from build123d import *

# Parameters (mm, degrees)
CYLINDER016_R     = 0.5
CYLINDER016_DEPTH = 10
CYLINDER014_R     = 2
CYLINDER014_DEPTH = 4
CYLINDER015_R     = 3
CYLINDER015_DEPTH = 10
BOX003_W          = 10
BOX003_H          = 10
BOX003_DEPTH      = 10
BOX004_W          = 2
BOX004_H          = 10
BOX004_DEPTH      = 10
BOX002_W          = 10
BOX002_H          = 10
BOX002_DEPTH      = 10
CYLINDER013_R     = 5
CYLINDER013_DEPTH = 10
CYLINDER012_R     = 5
CYLINDER012_DEPTH = 10


with BuildPart() as cylinder016:
    # Cylinder016 → Cylinder016 (new body)
    with BuildSketch(Plane(origin=(-5, 0, -7), x_dir=(0, 0, -1), z_dir=(1, 0, 0))):
        Circle(CYLINDER016_R)
    extrude(amount=CYLINDER016_DEPTH)


with BuildPart() as cylinder014:
    # Cylinder014 → Cylinder014 (new body)
    with BuildSketch(Plane(origin=(-2, -50, 1), x_dir=(0, 0, -1), z_dir=(1, 0, 0))):
        Circle(CYLINDER014_R)
    extrude(amount=CYLINDER014_DEPTH)


with BuildPart() as cylinder015:
    # Cylinder015 → Cylinder015 (new body)
    with BuildSketch(Plane(origin=(0, -50, -12), x_dir=(1, 0, 0), z_dir=(0, 0, 1))):
        Circle(CYLINDER015_R)
    extrude(amount=CYLINDER015_DEPTH)


with BuildPart() as cube003:
    # Box003 → Box003 (new body)
    with BuildSketch(Plane(origin=(-12, -55, -2), x_dir=(1, 0, 0), z_dir=(0, 0, 1))):
        with Locations((5, 5)):
            Rectangle(BOX003_W, BOX003_H)
    extrude(amount=BOX003_DEPTH)


with BuildPart() as cube004:
    # Box004 → Box004 (new body)
    with BuildSketch(Plane(origin=(-1, -55, -2), x_dir=(1, 0, 0), z_dir=(0, 0, 1))):
        with Locations((1, 5)):
            Rectangle(BOX004_W, BOX004_H)
    extrude(amount=BOX004_DEPTH)


with BuildPart() as cube002:
    # Box002 → Box002 (new body)
    with BuildSketch(Plane(origin=(2, -55, -2), x_dir=(1, 0, 0), z_dir=(0, 0, 1))):
        with Locations((5, 5)):
            Rectangle(BOX002_W, BOX002_H)
    extrude(amount=BOX002_DEPTH)


with BuildPart() as cylinder013:
    # Cylinder013 → Cylinder013 (new body)
    with BuildSketch(Plane(origin=(0, -50, -10), x_dir=(1, 0, 0), z_dir=(0, 0, 1))):
        Circle(CYLINDER013_R)
    extrude(amount=CYLINDER013_DEPTH)


with BuildPart() as sphere004:
    # Sphere004 → Sphere004 (revolve)
    with BuildSketch(Plane.XZ.offset(50)):
        with BuildLine():
            ThreePointArc((5, 0), (3.535534, 3.535534), (0, 5))
            Line((0, 5), (0, 0))
            Line((0, 0), (5, 0))
        make_face()
    revolve(axis=Axis((0, -50, 0), (0, 0, 1)))


with BuildPart() as cut013:
    # Cylinder012 → Cylinder012 (new body)
    with BuildSketch(Plane(origin=(0, -50, -7), x_dir=(1, 0, 0), z_dir=(0, 0, 1))):
        Circle(CYLINDER012_R)
    extrude(amount=CYLINDER012_DEPTH)

    # Common002: intersect Sphere004
    add(sphere004.part, mode=Mode.INTERSECT)

    # Fusion004: union Cylinder013
    add(cylinder013.part)

    # Cut009: cut Cube002
    add(cube002.part, mode=Mode.SUBTRACT)

    # Cut010: cut Cube004
    add(cube004.part, mode=Mode.SUBTRACT)

    # Cut011: cut Cube003
    add(cube003.part, mode=Mode.SUBTRACT)

    # Cut012: cut Cylinder015
    add(cylinder015.part, mode=Mode.SUBTRACT)

    # Fusion005: union Cylinder014
    add(cylinder014.part)


with BuildPart() as cut013_1:
    # Fusion005001 placement: moved
    add(cut013.part.moved(Location((0, 50, -8.5))))

    # Cut013: cut Cylinder016
    add(cylinder016.part, mode=Mode.SUBTRACT)


with BuildPart() as cut013_2:
    # Cut013 placement: moved
    add(cut013_1.part.moved(Location((0, 0, -18.5))))


solid = cut013_2.part
Check sheet for the modelled part. Datum: model origin and axes. Units: mm. A direction names the side the tool comes from. Round coordinates to 2 decimals unless told otherwise and drop trailing zeros. Write each loop counter-clockwise with the first axis right and the second up, starting at its lowest first coordinate (ties: lowest second). Pieces come first, ordered by that corner, then holes. Notation, with made-up numbers: (-34.5, 52.25) - (21.5, 52.25) arc R29 ccw to (21.5, 90.25) - close; hole circle Ø7 at (38, 87.5). An arc over 180 degrees is marked (long way). Return JSON: item names as keys, results as strings.
Q1. Access from +Z, -Z, +X, -X, +Y, -Y to the whole of each face (thin tool, end or side, straight path). Record for faces 4 (the cylindrical face through (-2.21, 2.03, -33.06)), 5 (the flat face through (3.5, 0.1, -29)), 6 (the flat face through (0, -4, -29)), 7 (the cylindrical face through (0, 2, -26)), 8 (the flat face through (-4, 0, -29)).
Returned:
{"face 4": "-Z", "face 5": "+Z, +X, +Y, -Y", "face 6": "+Z, +Y, -Y", "face 7": "none", "face 8": "+Z, -X, +Y, -Y"}
Q2. Cross-section at D-D (z = -27.5). Record the boundary of the cut face in (x, y), then the cut area to 3 significant figures.
Returned:
{"outline": "(-2, -4.58) arc R5 ccw to (-1, -4.9) - (-1, -1.32) - (1, -1.32) - (1, -4.9) arc R5 ccw to (2, -4.58) - (2, 4.58) arc R5 ccw to (1, 4.9) - (1, 1.32) - (-1, 1.32) - (-1, 4.9) arc R5 ccw to (-2, 4.58) - close", "area": "24.3 mm²"}
Q3. Depth check by flat-ended pin: P1, Ø1.5, axis at x = 3, y = 1, coming from the +Z side; P2, Ø0.5, axis at x = -1.5, y = -1, coming from the -Z side; P3, Ø2.5, axis at y = 1.5, z = -27.5, coming from the -X side. Enter the tip coordinate at first touch or a pass-through.
Returned:
{"P1": "stops at z = -29", "P2": "stops at z = -29", "P3": "stops at x = -2"}
Q4. Scan lines: L1, parallel to X at y = -1.75, z = -27.25; L2, parallel to Z at x = -1.15, y = 0; L3, parallel to Z at x = -0.05, y = 0. Record each from-to range of solid material in increasing order. Write a range as from..to.
Returned:
{"L1": "x = -2..-1, 1..2", "L2": "z = -29..-26, -25..-24", "L3": "z = -28..-26, -25..-24"}
Q5. Cross-section at C-C (x = -2.5). Record the boundary of the cut face in (y, z), then the cut area to 3 significant figures.
Returned:
{"outline": "(-4.33, -37) - (-1.66, -37) - (-1.66, -29) - (-4.33, -29) - close; (1.66, -37) - (4.33, -37) - (4.33, -29) - (1.66, -29) - close", "area": "42.7 mm²"}
Q6. Cross-section at A-A (x = 0). Record the boundary of the cut face in (y, z), then the cut area to 3 significant figures.
Returned:
{"outline": "(-5, -37) - (-3, -37) - (-3, -29) - (-5, -29) - close; circle Ø4 at (0, -26); (3, -37) - (5, -37) - (5, -29) - (3, -29) - close; hole circle Ø1 at (0, -25.5)", "area": "43.8 mm²"}
Q7. Cross-section at B-B (z = -31.5). Record the boundary of the cut face in (x, y), then the cut area to 3 significant figures.
Returned:
{"outline": "circle Ø10 at (0, 0); hole circle Ø6 at (0, 0)", "area": "50.3 mm²"}
Q8. Draft check along X on faces 1 (the flat face through (2, 0, -27)), 2 (the flat face through (-0.1, -3.3, -37)), 3 (the flat face through (0, 4, -29)). Enter one of: released by +X, released by -X, zero draft, split by the parting line, or undercut.
Returned:
{"face 1": "released by +X", "face 2": "zero draft", "face 3": "undercut"}
